Geometry: final body of the model. Coordinates: model frame, mm. A direction names the side the tool comes from. Coordinates: 2 decimals unless noted, no trailing zeros. Order: outer loops, then holes, each group sorted by start corner. A loop starts at its lowest first (then second) coordinate and runs counter-clockwise, first axis right, second up. Notation, with made-up numbers: (-24, -22.75) -> (-3, -22.75) arc R16 cw to (-3, 1.25) -> close; hole circle Ø10 at (81, 50). An arc over 180 degrees is marked (long way). Answer in a Markdown table with one row per item. Add a question column.
1) Contact query for flat-ended pins moving along their axis: P1, Ø6.5, axis at x = 6.5, y = -12, coming from the +Z side; P2, Ø6.5, axis at x = -24, y = -12.01, coming from the -Z side; P3, Ø5.5, axis at x = -8.5, z = 9.5, coming from the -Y side; P4, Ø2, axis at x = -8, z = 2.5, coming from the -Y side. Output: stop coordinate, or through.
2) Pull-direction query (Y, two-part tool) for faces 6 (the face through (-8, -10, 2)), 7 (the face through (-24.43, -13.96, 1.97)), 8 (the face through (-23.912, -16.005, 1.972)); classes: +Y half, -Y half, draft (parallel to the pull), parting line (faces both ways), or undercut.
3) Section query A-A on y = -0.85. Return the cut outline in (x, z), then the cut area to 3 significant figures.
4) Ray query, line 1 (Y direction, x = -4, z = 2.1); line 2 (X direction, y = -7, z = 7.25); line 3 (Y direction, x = 0, z = 9). Return the intervals inside material, ascending. Write a range as from..to.
5) Set-up query: faces 1 (the face through (11, -3.2, 6)), 2 (the face through (0, -4, 0)), 3 (the face through (11, 4, 5)), 4 (the face through (0, 7, 5)), 5 (the face through (-14, -8.006, 2)). Return all of +Z, -Z, +X, -X, +Y, -Y with unobstructed straight access to the full face (end or side cutting, diameter ignored); none if empty.
6) Section query B-B on x = 24. Return the cut outline in (y, z).
7) Section query C-C on x = 4. Return the cut outline in (y, z).
8) Section query D-D on y = -4. Return the cut outline in (x, z).
```python
from build123d import *

# Parameters (mm, degrees)
SCHIZZO1_W                   = 60
SCHIZZO1_H                   = 30
ESTRUSIONE_ESTRUSIONE1_DEPTH = 5
SCHIZZO2_W                   = 60
SCHIZZO2_H                   = 8
ESTRUSIONE_ESTRUSIONE2_DEPTH = 20
SCHIZZO3_R                   = 5
TAGLIO_ESTRUSIONE1_DEPTH     = 8
RACCORDO1_R                  = 20
SCHIZZO4_W                   = 60
SCHIZZO4_H                   = 15
ESTRUSIONE_ESTRUSIONE3_DEPTH = 10
SCHIZZO6_R                   = 8
TAGLIO_ESTRUSIONE2_DEPTH     = 15
SCHIZZO8_W                   = 60
SCHIZZO8_H                   = 4.7
ESTRUSIONE_ESTRUSIONE4_DEPTH = 10
SCHIZZO9_R                   = 6.3
TAGLIO_ESTRUSIONE3_DEPTH     = 5
SCHIZZO10_R                  = 2
TAGLIO_ESTRUSIONE4_DEPTH     = 16
SCHIZZO11_W                  = 60
SCHIZZO11_H                  = 8
TAGLIO_ESTRUSIONE5_DEPTH     = 25
SCHIZZO14_W                  = 60
SCHIZZO14_H                  = 5
TAGLIO_ESTRUSIONE7_DEPTH     = 7
SCHIZZO12_R                  = 2
ESTRUSIONE_ESTRUSIONE5_DEPTH = 4
SCHIZZO17_W                  = 60
SCHIZZO17_H                  = 15
TAGLIO_ESTRUSIONE9_DEPTH     = 3


with BuildPart() as part:
    # Schizzo1 → Estrusione-Estrusione1 (new body)
    with BuildSketch(Plane.XY):
        Rectangle(SCHIZZO1_W, SCHIZZO1_H)
    extrude(amount=ESTRUSIONE_ESTRUSIONE1_DEPTH)

    # Schizzo2 → Estrusione-Estrusione2 (add)
    with BuildSketch(Plane.XY.offset(5)):
        with Locations((0, 11)):
            Rectangle(SCHIZZO2_W, SCHIZZO2_H)
    extrude(amount=ESTRUSIONE_ESTRUSIONE2_DEPTH)

    # Schizzo3 → Taglio-Estrusione1 (cut)
    with BuildSketch(Plane(origin=(0, 15, 0), x_dir=(1, 0, 0), z_dir=(0, 1, 0))):
        with Locations((11, -13)):
            Circle(SCHIZZO3_R)
        with Locations((-11, -13)):
            Circle(SCHIZZO3_R)
    extrude(amount=-TAGLIO_ESTRUSIONE1_DEPTH, mode=Mode.SUBTRACT)

    # Raccordo1
    raccordo1_edges = [part.edges().sort_by_distance(p)[0] for p in [
        (30, 11, 25),
        (-30, 11, 25),
    ]]
    fillet(raccordo1_edges, radius=RACCORDO1_R)

    # Schizzo4 → Estrusione-Estrusione3 (add)
    with BuildSketch(Plane.XY.offset(5)):
        with Locations((0, -0.5)):
            Rectangle(SCHIZZO4_W, SCHIZZO4_H)
    extrude(amount=ESTRUSIONE_ESTRUSIONE3_DEPTH)

    # Schizzo6 → Taglio-Estrusione2 (cut)
    with BuildSketch(Plane.XZ.offset(8)):
        with Locations((-11, 13)):
            Circle(SCHIZZO6_R)
        with Locations((11, 13)):
            Circle(SCHIZZO6_R)
    extrude(amount=-TAGLIO_ESTRUSIONE2_DEPTH, mode=Mode.SUBTRACT)

    # Schizzo8 → Estrusione-Estrusione4 (add)
    with BuildSketch(Plane.XY.offset(15)):
        with Locations((0, -0.85)):
            Rectangle(SCHIZZO8_W, SCHIZZO8_H)
    extrude(amount=-ESTRUSIONE_ESTRUSIONE4_DEPTH)

    # Schizzo9 → Taglio-Estrusione3 (cut)
    with BuildSketch(Plane.XZ.offset(3.2)):
        with Locations((-11, 13)):
            Circle(SCHIZZO9_R)
        with Locations((11, 13)):
            Circle(SCHIZZO9_R)
    extrude(amount=-TAGLIO_ESTRUSIONE3_DEPTH, mode=Mode.SUBTRACT)

    # Schizzo10 → Taglio-Estrusione4 (cut, through all)
    with BuildSketch(Plane.XY.offset(15)):
        with Locations((0, -0.85)):
            Circle(SCHIZZO10_R)
        with Locations((24, -0.85)):
            Circle(SCHIZZO10_R)
        with Locations((-24, -0.85)):
            Circle(SCHIZZO10_R)
    extrude(amount=-TAGLIO_ESTRUSIONE4_DEPTH, mode=Mode.SUBTRACT)

    # Schizzo11 → Taglio-Estrusione5 (cut)
    with BuildSketch(Plane(origin=(0, 0, 0), x_dir=(-1, 0, 0), z_dir=(0, 0, -1))):
        with Locations((0, 11)):
            Rectangle(SCHIZZO11_W, SCHIZZO11_H)
    extrude(amount=-TAGLIO_ESTRUSIONE5_DEPTH, mode=Mode.SUBTRACT)

    # Schizzo14 → Taglio-Estrusione7 (cut)
    with BuildSketch(Plane.XZ.offset(15)):
        with Locations((0, 2.5)):
            Rectangle(SCHIZZO14_W, SCHIZZO14_H)
    extrude(amount=-TAGLIO_ESTRUSIONE7_DEPTH, mode=Mode.SUBTRACT)

    # Schizzo12 → Estrusione-Estrusione5 (add)
    with BuildSketch(Plane.XY):
        with BuildLine():
            Line((-28, -12.006435696), (-28, -5.256435696))
            Line((-28, -5.256435696), (28, -5.256435696))
            Line((28, -5.256435696), (28, -12.006435696))
            ThreePointArc((28, -12.006435696), (24, -16.006435696), (20, -12.006435696))
            Line((20, -12.006435696), (20, -8.006435696))
            Line((20, -8.006435696), (8, -8.006435696))
            Line((8, -8.006435696), (8, -12.006435696))
            ThreePointArc((8, -12.006435696), (4, -16.006435696), (0, -12.006435696))
            ThreePointArc((0, -12.006435696), (-4, -16.006435696), (-8, -12.006435696))
            Line((-8, -12.006435696), (-8, -8.006435696))
            Line((-8, -8.006435696), (-20, -8.006435696))
            Line((-20, -8.006435696), (-20, -12.006435696))
            ThreePointArc((-20, -12.006435696), (-24, -16.006435696), (-28, -12.006435696))
        make_face()
        with Locations((24, -12.006435696)):
            Circle(SCHIZZO12_R, mode=Mode.SUBTRACT)
        with Locations((-24, -12.006435696)):
            Circle(SCHIZZO12_R, mode=Mode.SUBTRACT)
        with Locations((4, -12.006435696)):
            Circle(SCHIZZO12_R, mode=Mode.SUBTRACT)
        with Locations((-4, -12.006435696)):
            Circle(SCHIZZO12_R, mode=Mode.SUBTRACT)
    extrude(amount=ESTRUSIONE_ESTRUSIONE5_DEPTH)

    # Schizzo17 → Taglio-Estrusione9 (cut)
    with BuildSketch(Plane.XY.offset(15)):
        with Locations((0, -0.5)):
            Rectangle(SCHIZZO17_W, SCHIZZO17_H)
    extrude(amount=-TAGLIO_ESTRUSIONE9_DEPTH, mode=Mode.SUBTRACT)


solid = part.part
```
Result:
| question | item | result |
|---|---|---|
| 1 | P1 | z = 4 |
| 1 | P2 | z = 0 |
| 1 | P3 | y = -3.2 |
| 1 | P4 | y = -14.65 |
| 2 | face 6 | draft |
| 2 | face 7 | undercut |
| 2 | face 8 | -Y half |
| 3 | outline | (-30, 0) -> (-26, 0) -> (-26, 12) -> (-30, 12) -> close; (-22, 0) -> (-2, 0) -> (-2, 12) -> (-4.78, 12) arc R6.3 cw to (-17.22, 12) -> (-22, 12) -> close; (2, 0) -> (22, 0) -> (22, 12) -> (17.22, 12) arc R6.3 cw to (4.78, 12) -> (2, 12) -> close; (26, 0) -> (30, 0) -> (30, 12) -> (26, 12) -> close |
| 3 | area | 476 mm2 |
| 4 | line 1 | -16.01..-14.01, -10.01..7 |
| 4 | line 2 | -30..-16.56, -5.44..5.44, 16.56..30 |
| 4 | line 3 | -8..-2.85, 1.15..7 |
| 5 | face 1 | +Z, -Y |
| 5 | face 2 | -Z, +X, -X, +Y, -Y |
| 5 | face 3 | +Z, +Y |
| 5 | face 4 | +Z, -Z, +X, -X, +Y |
| 5 | face 5 | +Z, -Z, -Y |
| 6 | outline | (-16.01, 0) -> (-14.01, 0) -> (-14.01, 4) -> (-16.01, 4) -> close; (-10.01, 0) -> (-2.85, 0) -> (-2.85, 12) -> (-8, 12) -> (-8, 4) -> (-10.01, 4) -> close; (1.15, 0) -> (7, 0) -> (7, 12) -> (1.15, 12) -> close |
| 7 | outline | (-16.01, 0) -> (-14.01, 0) -> (-14.01, 4) -> (-16.01, 4) -> close; (-10.01, 0) -> (7, 0) -> (7, 9.13) -> (1.5, 9.13) -> (1.5, 12) -> (-3.2, 12) -> (-3.2, 9.13) -> (-8, 9.13) -> (-8, 4) -> (-10.01, 4) -> close |
| 8 | outline | (-30, 0) -> (30, 0) -> (30, 12) -> (18.94, 12) arc R8 cw to (3.06, 12) -> (-3.06, 12) arc R8 cw to (-18.94, 12) -> (-30, 12) -> close |
